```python
from build123d import *

# Parameters (mm, degrees)
BOSS_EXTRUDE1_DEPTH   = 3.175
SKETCH2_R             = 3.7703125
CUT_EXTRUDE1_DEPTH    = 4.1750001
SKETCH4_R             = 6.096
SKETCH4_R_2           = 1.905
CUT_EXTRUDE2_DEPTH    = 4.1750001
F_6_CLEARANCE_HOLE1_D = 4.3053
SKETCH7_R             = 1.190625
CUT_EXTRUDE3_DEPTH    = 4.1750001


with BuildPart() as part:
    # Sketch1 → Boss-Extrude1 (new body)
    with BuildSketch(Plane.XY):
        with BuildLine():
            Line((-51.59375, 5.432306697), (-87.3125, 5.432306697))
            add(Edge.make_bspline(
                [(-87.3125, 5.432306697), (-88.9, 5.432306697), (-88.9, 3.742924483)],
                knots=[3.141592654, 3.141592654, 3.141592654, 4.71238898, 4.71238898, 4.71238898], degree=2, weights=[1, 0.707106781, 1]))
            Line((-88.9, 3.742924483), (-88.9, -39.099808459))
            add(Edge.make_bspline(
                [(-88.9, -39.099808459), (-88.9, -40.789190673), (-87.3125, -40.789190673)],
                knots=[1.570796327, 1.570796327, 1.570796327, 3.141592654, 3.141592654, 3.141592654], degree=2, weights=[1, 0.707106781, 1]))
            Line((-87.3125, -40.789190673), (87.3125, -40.789190673))
            add(Edge.make_bspline(
                [(87.3125, -40.789190673), (88.9, -40.789190673), (88.9, -39.099808459)],
                knots=[3.141592654, 3.141592654, 3.141592654, 4.71238898, 4.71238898, 4.71238898], degree=2, weights=[1, 0.707106781, 1]))
            Line((88.9, -39.099808459), (88.9, 3.742924483))
            add(Edge.make_bspline(
                [(88.9, 3.742924483), (88.9, 5.432306697), (87.3125, 5.432306697)],
                knots=[1.570796327, 1.570796327, 1.570796327, 3.141592654, 3.141592654, 3.141592654], degree=2, weights=[1, 0.707106781, 1]))
            Line((87.3125, 5.432306697), (51.59375, 5.432306697))
            add(Edge.make_bspline(
                [(50.8, 6.276997804), (50.8, 5.432306697), (51.59375, 5.432306697)],
                knots=[4.71238898, 4.71238898, 4.71238898, 6.283185307, 6.283185307, 6.283185307], degree=2, weights=[1, 0.707106781, 1]))
            Line((50.8, 6.276997804), (50.8, 32.394846829))
            add(Edge.make_bspline(
                [(50.8, 32.394846829), (50.8, 34.084229043), (49.2125, 34.084229043)],
                knots=[4.71238898, 4.71238898, 4.71238898, 6.283185307, 6.283185307, 6.283185307], degree=2, weights=[1, 0.707106781, 1]))
            Line((49.2125, 34.084229043), (-49.2125, 34.084229043))
            add(Edge.make_bspline(
                [(-49.2125, 34.084229043), (-50.8, 34.084229043), (-50.8, 32.394846829)],
                knots=[0, 0, 0, 1.570796327, 1.570796327, 1.570796327], degree=2, weights=[1, 0.707106781, 1]))
            Line((-50.8, 32.394846829), (-50.8, 6.276997804))
            add(Edge.make_bspline(
                [(-51.59375, 5.432306697), (-50.8, 5.432306697), (-50.8, 6.276997804)],
                knots=[0, 0, 0, 1.570796327, 1.570796327, 1.570796327], degree=2, weights=[1, 0.707106781, 1]))
        make_face()
    extrude(amount=BOSS_EXTRUDE1_DEPTH)

    # Sketch2 → Cut-Extrude1 (cut, through all)
    with BuildSketch(Plane.XY.offset(3.175)):
        with Locations((42.8625, -15.909796167)):
            Circle(SKETCH2_R)
        with Locations((-15.875, -15.909796167)):
            Circle(SKETCH2_R)
        with Locations((-74.6125, -15.909796167)):
            Circle(SKETCH2_R)
        with Locations((34.29, 13.617703833)):
            Circle(SKETCH2_R)
    extrude(amount=-CUT_EXTRUDE1_DEPTH, mode=Mode.SUBTRACT)

    # Sketch4 → Cut-Extrude2 (cut, through all)
    with BuildSketch(Plane.XY.offset(3.175)):
        with Locations((73.025, -15.909796167)):
            Circle(SKETCH4_R)
        with Locations((12.7, -15.909796167)):
            Circle(SKETCH4_R)
        with Locations((-44.45, -15.909796167)):
            Circle(SKETCH4_R)
        with Locations((-24.13, 13.617703833)):
            Circle(SKETCH4_R)
        with Locations((6.35, 13.617703833)):
            Circle(SKETCH4_R)
        with Locations((73.025, -25.434796167)):
            Circle(SKETCH4_R_2)
        with Locations((12.7, -25.434796167)):
            Circle(SKETCH4_R_2)
        with Locations((-44.45, -25.434796167)):
            Circle(SKETCH4_R_2)
        with Locations((6.35, 4.092703833)):
            Circle(SKETCH4_R_2)
        with Locations((-24.13, 4.092703833)):
            Circle(SKETCH4_R_2)
    extrude(amount=-CUT_EXTRUDE2_DEPTH, mode=Mode.SUBTRACT)

    # #6 Clearance Hole1 (through all)
    with Locations(Plane.XY.offset(3.175)):
        with Locations((-45.72, 27.270203833), (16.51, 27.270203833), (21.59, 19.015203833), (57.15, -8.924796167), (57.15, -31.149796167), (-60.96, -31.149796167), (-60.96, -8.924796167)):
            Hole(F_6_CLEARANCE_HOLE1_D / 2)

    # Sketch7 → Cut-Extrude3 (cut, through all)
    with BuildSketch(Plane.XY.offset(3.175)):
        with Locations((42.967003171, -9.910706312)):
            Circle(SKETCH7_R)
        with Locations((-15.773980268, -10.110675974)):
            Circle(SKETCH7_R)
        with Locations((-74.507996829, -9.910706312)):
            Circle(SKETCH7_R)
        with Locations((34.394503171, 19.616793688)):
            Circle(SKETCH7_R)
    extrude(amount=-CUT_EXTRUDE3_DEPTH, mode=Mode.SUBTRACT)


solid = part.part
```
Part model, mm, in its own coordinate system. A direction names the side the tool comes from. Give positions to 0.01 mm unless a question says otherwise; leave off trailing zeros. Order: outer loops, then holes, each group sorted by start corner. A loop starts at its lowest first (then second) coordinate and runs counter-clockwise, first axis right, second up. Notation, with made-up numbers: M 5.25,28 L 50.25,28 A31 ccw 50.25,67 Z; hole C -12.5,86 d1. An arc over 180 degrees is marked long. Use a Markdown table: item, result. Add a question column.
(1) Saw through at B-B, the plane x = 21. Give the cut face in (y, z) (3 decimals), and give its area (3 significant figures).
(2) Saw through at A-A, the plane x = -24.13. Give the cut face in (y, z) (3 decimals), and give its area (3 significant figures).
(3) Drop flat-ended pins along their axis: P1, Ø1.6, axis at y = 24.5, z = 2, coming from the -X side; P2, Ø1.5, axis at x = -55.5, z = 2.5, coming from the +Y side. Give the stop position or say it passes through.
(4) Mould opens along X. For faces 3 (the face through (30.523, 13.783, 1.61)), 4 (the face through (-1, -11, 0)), 5 (the face through (-88.9, -17, 2)) say: +X half, -X half, draft (parallel to the pull), parting line (faces both ways), or undercut.
(5) 3-axis set-ups, long thin cutter, end or side, ignore diameter. For faces 1 (the face through (70, 5.432, 2)), 2 (the face through (-14.135, -19.255, 1.61)): which of +Z, -Z, +X, -X, +Y, -Y reach the whole face in a straight line?
(6) Probe line 1 along Y through (x, z) = (6, 1.6); line 2 along X through (y, z) = (-27, 1.55); line 3 along X through (y, z) = (9.5, 0.2). List the from-to ranges inside material, lowest first. Write a range as [from, to].
(7) Saw through at C-C, the plane z = 1.9. Give the number of separate pieces and of enclosed holes in the cut face, and give its area (3 significant figures).
Answer key:
| question | item | result |
|---|---|---|
| 1 | outline | M -40.789,0 L 16.945,0 L 16.945,3.175 L -40.789,3.175 Z; M 21.085,0 L 34.084,0 L 34.084,3.175 L 21.085,3.175 Z |
| 1 | area | 225 mm^2 |
| 2 | outline | M -40.789,0 L 2.188,0 L 2.188,3.175 L -40.789,3.175 Z; M 5.998,0 L 7.522,0 L 7.522,3.175 L 5.998,3.175 Z; M 19.714,0 L 34.084,0 L 34.084,3.175 L 19.714,3.175 Z |
| 2 | area | 187 mm^2 |
| 3 | P1 | x = -50.8 |
| 3 | P2 | y = 5.43 |
| 4 | face 3 | undercut |
| 4 | face 4 | draft |
| 4 | face 5 | -X half |
| 5 | face 1 | +Z, -Z, +X, +Y |
| 5 | face 2 | +Z, -Z |
| 6 | line 1 | [-40.79, 2.22], [5.97, 7.53], [19.7, 34.08] |
| 6 | line 2 | [-88.9, -45.54], [-43.36, 11.61], [13.79, 71.94], [74.11, 88.9] |
| 6 | line 3 | [-50.8, -28.63], [-19.63, 1.85], [10.85, 50.8] |
| 7 | separate pieces | 1 |
| 7 | enclosed holes | 25 |
| 7 | area | 10,200 mm^2 |
